Could you check a few things on this model? Use its own coordinates, in mm. Face numbers are marked on the shaded views. Give positions to 0.01 mm unless a question says otherwise; leave off trailing zeros. Loops run counter-clockwise (first coordinate to the right, second up) from the corner with the lowest first, then second, coordinate; pieces in that order, holes last. Notation, with made-up numbers: (85.25, 16) - (139.25, 16) arc R16 cw to (139.25, 27) - close; hole circle Ø8 at (43.25, 63.25). An arc over 180 degrees is marked (long way). Write each question's results on one line, items separated by ' | '. Start each with the question number.
Autodesk Inventor part; units mm, degrees
ref_plane "YZ Plane" through (0, 0, 0) normal (1, 0, 0) x (0, 1, 0)
ref_plane "XZ Plane" through (0, 0, 0) normal (0, 1, 0) x (-1, 0, 0)
ref_plane "XY Plane" through (0, 0, 0) normal (0, 0, 1) x (1, 0, 0)
sketch "Эскиз1" plane through (0, 0, 0) normal (0, 0, 1) x (1, 0, 0)
  line L0 (0, 26) -> (0, -26)
  line L1 (12.573, 26) -> (13.8571, 26)
  line L2 (14.125, 25) -> (14.125, -25)
  line L3 (13.8571, -26) -> (12.573, -26)
  line L4 (12.573, -26) -> (12.573, 26)
  line L5 (14.125, 25) -> (13.8571, 26)
  line L6 (14.125, -25) -> (13.8571, -26)
  point P0 (0, 0)
  point P1 (0, 0)
  point P2 (14.125, -26)
  point P3 (14.125, 26)
  dimension "d0" = 52
  dimension "d1" = 28.25
  dimension "d2" = 25.146
  dimension "d3" = 1
  dimension "d4" = 15
  dimension "d5" = 1
  dimension "d6" = 15
revolve "Вращение1" add sketch "Эскиз1" angle 360 about axis through (0, 26, 0) along (0, -1, 0)
sketch "Эскиз2" plane through (0, 26, 0) normal (0, 1, 0) x (1, 0, 0)
  line L0 (12.5107, 1.25) -> (12.8107, 1.25)
  line L1 (12.8107, 1.25) -> (12.8107, -1.25)
  line L2 (12.8107, -1.25) -> (12.5107, -1.25)
  line L3 (12.5107, -1.25) -> (12.5107, 1.25)
  circle A0 centre (0, 0) radius 12.573
  point P0 (0, 0)
  point P1 (12.5107, 0)
  dimension "d8" = 2.5
  dimension "d10" = 0.3
extrude "Выдавливание1" cut sketch "Эскиз2" against normal through all contours A0 L3 | L0 L1 L2 A0 picked at (12.5222, -0.278)
pattern_circular "Круговой массив1" count 3 over 360 about axis through (0, 0, 0) along (0, -1, 0) of "Выдавливание1"
equation "\"d6\" = d4"
properties part number "75. Втулка блока заднего хода"
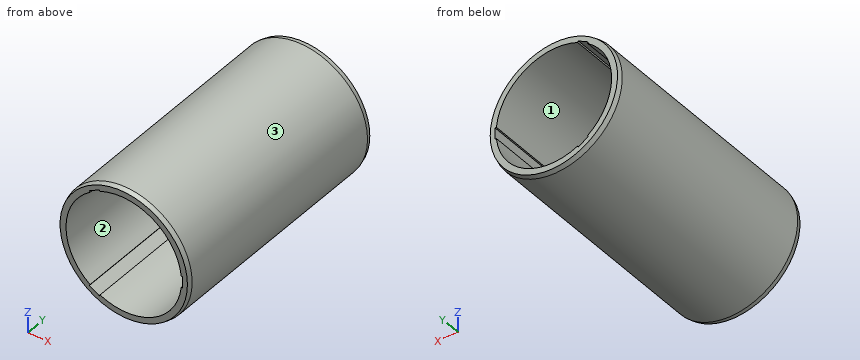
Q1. I need wall thicknesses on L1, parallel to Z at x = 0.5, y = 21.5; L2, parallel to X at y = -10, z = -3.25; L3, parallel to X at y = -22, z = 6. Which ranges of each line are inside material? Lowest first, please. Write a range as from..to.
Q2. I'm going to push flat-ended pins straight in: pin 1 Ø1.5 at (x, y) = (10, 10) entering from -Z; pin 2 Ø8 at (x, z) = (-2, -10.5) entering from +Y; pin 3 Ø4 at (y, z) = (-5, -10) entering from +X; pin 4 Ø2 at (y, z) = (13, -5) entering from +X. Where does each tip first touch, or does it pass through?
Q3. I want a section at C-C, the plane y = -7.5. List the corners of the cut face in (x, z) for me (3 decimals).
Q4. If we mould it in two halves opening along X, with no side actions, what happens to the marked faces 1, 2 and 3? For each: +X half, -X half, draft (parallel to the pull), parting line (faces both ways), or undercut.
Q5. I want a section at B-B, the plane z = 0. List the corners of the cut face in (x, y) for me (3 decimals).
Q6. I want a section at A-A, the plane x = 0. List the corners of the cut face in (y, z) for me (3 decimals).
Conclusion:
1) L1: -14.12..-12.56, 12.56..14.12 | L2: -13.75..-12.15, 12.15..13.75 | L3: -12.79..-11.05, 11.05..12.79
2) pin 1: z = -10.67 | pin 2: y = 26 | pin 3: x = 11.64 | pin 4: x = 13.55
3) outline: circle Ø28.25 at (0, 0); hole (-7.488, -10.469) - (-5.323, -11.719) - (-5.173, -11.46) arc R12.573 ccw to (12.511, -1.25) - (12.811, -1.25) - (12.811, 1.25) - (12.511, 1.25) arc R12.573 ccw to (-5.173, 11.46) - (-5.323, 11.719) - (-7.488, 10.469) - (-7.338, 10.21) arc R12.573 ccw to (-7.338, -10.21) - close
4) face 1: undercut | face 2: undercut | face 3: parting line
5) outline: (-14.125, -25) - (-13.857, -26) - (-12.573, -26) - (-12.573, 26) - (-13.857, 26) - (-14.125, 25) - close; (12.811, -26) - (13.857, -26) - (14.125, -25) - (14.125, 25) - (13.857, 26) - (12.811, 26) - close
6) outline: (-26, -13.857) - (-25, -14.125) - (25, -14.125) - (26, -13.857) - (26, -12.573) - (-26, -12.573) - close; (-26, 12.573) - (26, 12.573) - (26, 13.857) - (25, 14.125) - (-25, 14.125) - (-26, 13.857) - close
